from build123d import *

# Parameters (mm, degrees)
BOSS_EXTRUDE1_DEPTH = 70
SHELL1_T            = -3
SKETCH5_W           = 100
SKETCH5_H           = 80
CUT_EXTRUDE2_DEPTH  = 30
FILLET1_R           = 10
FILLET2_R           = 3


with BuildPart() as part:
    # Sketch3 → Boss-Extrude1 (new body)
    with BuildSketch(Plane(origin=(0, 0, 0), x_dir=(1, 0, 0), z_dir=(0, 1, 0))):
        Polygon((0, 199.904133626), (-141.353568474, 141.353568474), (-199.904133626, 0), (-141.353568474, -141.353568474), (0, -199.904133626), (141.353568474, -141.353568474), (199.904133626, 0), (141.353568474, 141.353568474), align=None)
    extrude(amount=BOSS_EXTRUDE1_DEPTH)

    # Shell1
    shell1_openings = [part.faces().sort_by_distance(p)[0] for p in [
        (0, 0, 0),
    ]]
    offset(amount=SHELL1_T, openings=shell1_openings, kind=Kind.INTERSECTION)

    # Sketch5 → Cut-Extrude2 (cut)
    with BuildSketch(Plane(origin=(331, 0, 0), x_dir=(0, 0, -1), z_dir=(1, 0, 0))):
        with Locations((0, 40)):
            Rectangle(SKETCH5_W, SKETCH5_H)
    extrude(amount=-CUT_EXTRUDE2_DEPTH, mode=Mode.SUBTRACT)

    # Fillet1
    fillet1_edges = [part.edges().sort_by_distance(p)[0] for p in [
        (170.62885105, 70, -70.676784237),
        (70.676784237, 70, -170.62885105),
        (-70.676784237, 70, -170.62885105),
        (-170.62885105, 70, -70.676784237),
        (-170.62885105, 70, 70.676784237),
        (-70.676784237, 70, 170.62885105),
        (70.676784237, 70, 170.62885105),
        (170.62885105, 70, 70.676784237),
    ]]
    fillet(fillet1_edges, radius=FILLET1_R)

    # Fillet2
    fillet2_edges = [part.edges().sort_by_distance(p)[0] for p in [
        (69.52873394, 67, 167.857212453),
        (167.857212453, 67, 69.52873394),
        (167.857212453, 67, -69.52873394),
        (69.52873394, 67, -167.857212453),
        (-69.52873394, 67, -167.857212453),
        (-167.857212453, 67, -69.52873394),
        (-167.857212453, 67, 69.52873394),
        (-69.52873394, 67, 167.857212453),
    ]]
    fillet(fillet2_edges, radius=FILLET2_R)


solid = part.part
Verification items for the finished model (mm, model axes). A direction names the side the tool comes from. Coordinates: 2 decimals unless noted, no trailing zeros. Order: outer loops, then holes, each group sorted by start corner. A loop starts at its lowest first (then second) coordinate and runs counter-clockwise, first axis right, second up. Notation, with made-up numbers: (38, -39.5) -> (71, -39.5) arc R9 cw to (71, -23.5) -> close; hole circle Ø3 at (-14.75, 40.25). An arc over 180 degrees is marked (long way). Put each result on its own line as item: value. Start each with the question number.
1. Access from +Z, -Z, +X, -X, +Y, -Y to the whole of each face (thin tool, end or side, straight path). Record for faces 1 (the cylindrical face through (68.596, 66.993, -168.404)), 2 (the cylindrical face through (-68.228, 66.098, 167.47)).
2. Cross-section at A-A, the plane y = 27. Record the boundary of the cut face in (x, z), then the cut area to 3 significant figures.
3. Mould release check, pull along Z, two halves, no side actions. Record for faces 3 (the flat face through (-3, 70, -3)), 4 (the flat face through (71.666, 29.58, -170.219)), 5 (the cylindrical face through (168.404, 66.993, 68.596)), 6 (the cylindrical face through (70.175, 66.098, 166.664)): released by +Z, released by -Z, zero draft, split by the parting line, or undercut.
4. Go/stop test with flat-tipped pins: pin 1 Ø4 at (y, z) = (19, -57) entering from +X; pin 2 Ø6 at (y, z) = (7.5, 26) entering from +X; pin 3 Ø1 at (y, z) = (29, -154) entering from -X. Record where each tip stops, or that it passes through.
5. Material ranges on L1, parallel to X at y = 57.5, z = -8; L2, parallel to Y at x = 119.5, z = -102.5; L3, parallel to X at y = 34.5, z = -179.5, recorded low to high. Write a range as [from, to].
Computed:
1. face 1: -Z, +X, +Y
1. face 2: -Y
2. outline: (-199.9, 0) -> (-141.35, -141.35) -> (0, -199.9) -> (141.35, -141.35) -> (199.9, 0) -> (141.35, 141.35) -> (0, 199.9) -> (-141.35, 141.35) -> close; hole (-196.66, 0) -> (-139.06, -139.06) -> (0, -196.66) -> (139.06, -139.06) -> (196.66, 0) -> (139.06, 139.06) -> (0, 196.66) -> (-139.06, 139.06) -> close
2. area: 3,640 mm2
3. face 3: zero draft
3. face 4: released by -Z
3. face 5: released by +Z
3. face 6: undercut
4. pin 1: x = 177.12
4. pin 2: x = 190.38
4. pin 3: x = -112.03
5. L1: [-196.59, -193.34], [193.34, 196.59]
5. L2: [67, 70]
5. L3: [-49.26, -41.42], [41.42, 49.26]
